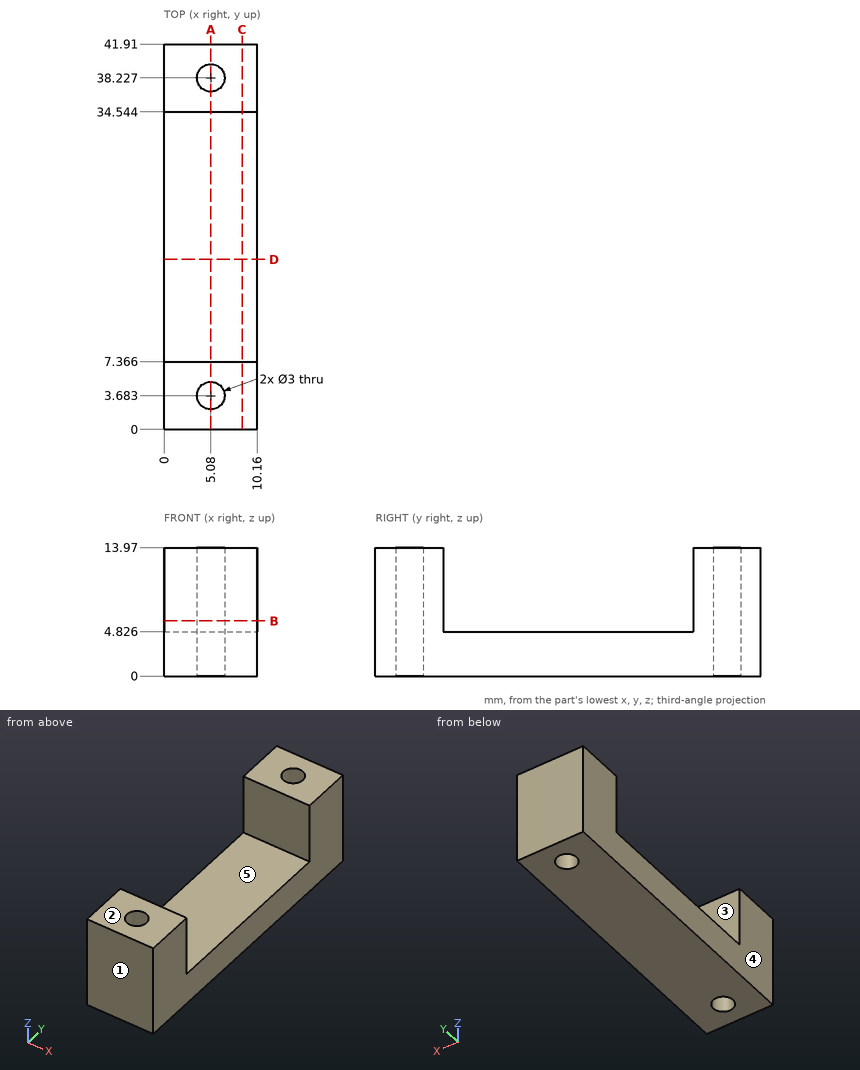
Input: dimensioned drawing with shaded views. Units: mm. Origin: part minimum x, y, z. A direction names the side the tool comes from. Round coordinates to 2 decimals unless told otherwise and drop trailing zeros. Loops run counter-clockwise (first coordinate to the right, second up) from the corner with the lowest first, then second, coordinate; pieces in that order, holes last.
1) Pull-direction query (Y, two-part tool) for the marked faces 1, 2 and 3; classes: released by +Y, released by -Y, zero draft, split by the parting line, or undercut.
Ans:
face 1: released by -Y
face 2: zero draft
face 3: undercut
2) Set-up query: the marked faces 4 and 5. Return all of +Z, -Z, +X, -X, +Y, -Y with unobstructed straight access to the full face (end or side cutting, diameter ignored); none if empty.
Ans:
face 4: +Z, -Z, -X, +Y, -Y
face 5: +Z, +X, -X
3) Pin query (flat end, axial travel): pin 1 (2 mm diameter, centred on x = 1, z = 5.5, fed in from -Y). Return the tip coordinate at first contact, or that it passes through.
Ans:
pin 1: stops at y = 0
4) Material intervals for line 1 (Y direction, x = 5.25, z = 9.75); line 2 (Y direction, x = 5.08, z = 4.5); line 3 (Y direction, x = 2.5, z = 7), sorted ascending.
Ans:
line 1: y = 0 to 2.19, 5.17 to 7.37, 34.54 to 36.74, 39.72 to 41.91
line 2: y = 0 to 2.18, 5.18 to 36.73, 39.73 to 41.91
line 3: y = 0 to 7.37, 34.54 to 41.91
5) Section query D-D on y = 18.5. Return the cut outline in (x, z).
Ans:
outline: (0, 0) - (10.16, 0) - (10.16, 4.83) - (0, 4.83) - close
6) Section query A-A on x = 5.08. Return the cut outline in (y, z).
Ans:
outline: (0, 0) - (2.18, 0) - (2.18, 13.97) - (0, 13.97) - close; (5.18, 0) - (36.73, 0) - (36.73, 13.97) - (34.54, 13.97) - (34.54, 4.83) - (7.37, 4.83) - (7.37, 13.97) - (5.18, 13.97) - close; (39.73, 0) - (41.91, 0) - (41.91, 13.97) - (39.73, 13.97) - close
7) Section query B-B on z = 6. Return the cut outline in (x, y).
Ans:
outline: (0, 0) - (10.16, 0) - (10.16, 7.37) - (0, 7.37) - close; (0, 34.54) - (10.16, 34.54) - (10.16, 41.91) - (0, 41.91) - close; hole circle Ø3 at (5.08, 3.68); hole circle Ø3 at (5.08, 38.23)
8) Section query C-C on x = 8.5. Return the cut outline in (y, z), plus the area to 3 significant figures.
Ans:
outline: (0, 0) - (41.91, 0) - (41.91, 13.97) - (34.54, 13.97) - (34.54, 4.83) - (7.37, 4.83) - (7.37, 13.97) - (0, 13.97) - close
area: 337 mm2
